Geometry: see drawing. Coordinates: mm, zero at the bounding-box minimum. Round coordinates to 2 decimals unless told otherwise and drop trailing zeros. Order: outer loops, then holes, each group sorted by start corner. A loop starts at its lowest first (then second) coordinate and runs counter-clockwise, first axis right, second up. Notation, with made-up numbers: (-37.5, 26) -> (-5.5, 26) arc R13 ccw to (-5.5, 50) -> close; hole circle Ø5 at (24.25, 63). An arc over 180 degrees is marked (long way). Use a Markdown table: item, result.
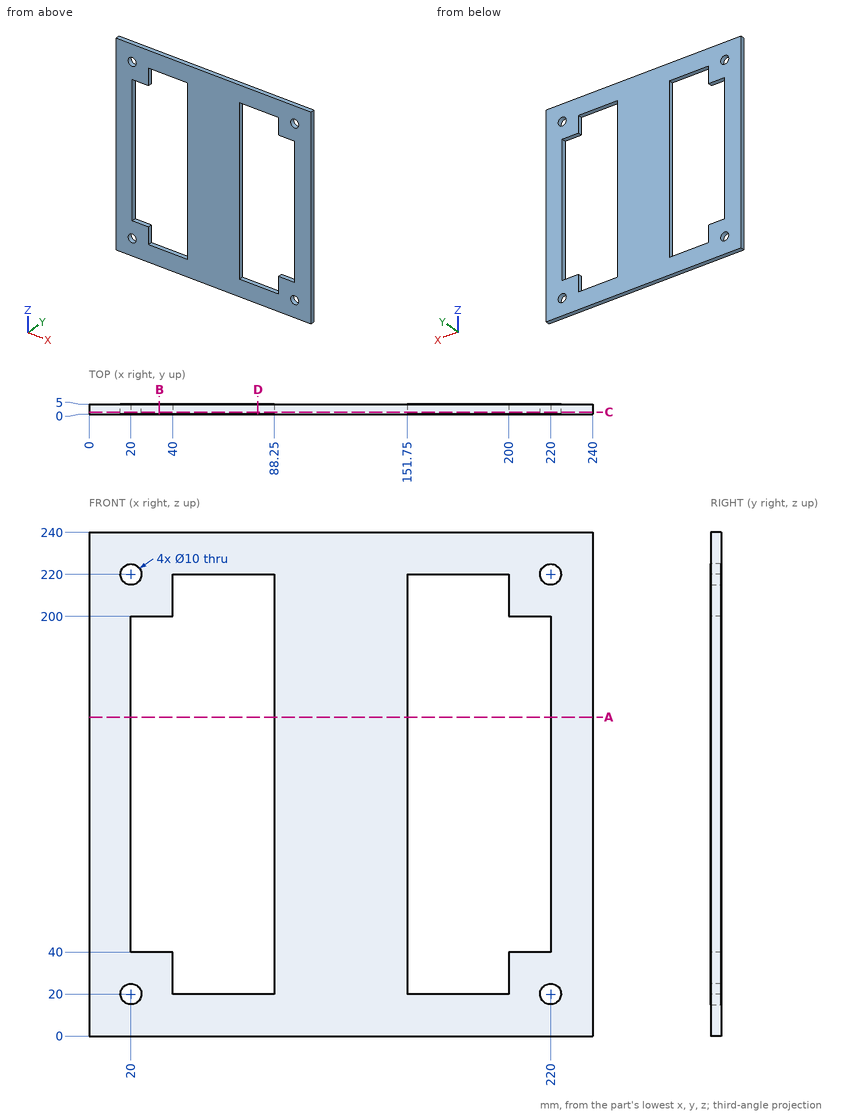
1) Ray query, probe 1 along X at (y, z) = (0.5, 211); probe 2 along X at (y, z) = (1.6, 175); probe 3 along Z at (x, y) = (67.5, 4.7). Return the intervals inside material, ascending.
Answer key:
| item | result |
|---|---|
| probe 1 | x = 0 to 40, 88.25 to 151.75, 200 to 240 |
| probe 2 | x = 0 to 20, 88.25 to 151.75, 220 to 240 |
| probe 3 | z = 0 to 20, 220 to 240 |
2) Cut plane D-D on x = 80.5. Return loops of the section in (y, z), and give its area (3 significant figures).
Answer key:
| item | result |
|---|---|
| outline | (0, 0) -> (5, 0) -> (5, 20) -> (0, 20) -> close; (0, 220) -> (5, 220) -> (5, 240) -> (0, 240) -> close |
| area | 200 mm^2 |
3) Cut plane A-A on z = 152. Return loops of the section in (x, y), and give its area (4 significant figures).
Answer key:
| item | result |
|---|---|
| outline | (0, 0) -> (20, 0) -> (20, 5) -> (0, 5) -> close; (88.25, 0) -> (151.75, 0) -> (151.75, 5) -> (88.25, 5) -> close; (220, 0) -> (240, 0) -> (240, 5) -> (220, 5) -> close |
| area | 517.5 mm^2 |
4) Cut plane C-C on y = 1.1. Return loops of the section in (x, z).
Answer key:
| item | result |
|---|---|
| outline | (0, 0) -> (240, 0) -> (240, 240) -> (0, 240) -> close; hole circle Ø10 at (20, 20); hole circle Ø10 at (20, 220); hole (20, 40) -> (40, 40) -> (40, 20) -> (88.25, 20) -> (88.25, 220) -> (40, 220) -> (40, 200) -> (20, 200) -> close; hole (151.75, 20) -> (200, 20) -> (200, 40) -> (220, 40) -> (220, 200) -> (200, 200) -> (200, 220) -> (151.75, 220) -> close; hole circle Ø10 at (220, 20); hole circle Ø10 at (220, 220) |
5) Contact query for a flat-ended pin moving along its axis: P1, Ø13, axis at x = 20, z = 220, coming from the -Y side. Output: stop coordinate, or through.
Answer key:
| item | result |
|---|---|
| P1 | stops at y = 0 |
6) Cut plane B-B on x = 33.5. Return loops of the section in (y, z).
Answer key:
| item | result |
|---|---|
| outline | (0, 0) -> (5, 0) -> (5, 40) -> (0, 40) -> close; (0, 200) -> (5, 200) -> (5, 240) -> (0, 240) -> close |
